from build123d import *

# Parameters (mm, degrees)
SKETCH_1_W          = 95.45
SKETCH_1_H          = 35.35
SKETCH_1_R          = 2
EXTRUDE_1_DEPTH     = 5
SKETCH_2_R          = 2
CUT_EXTRUDE_1_DEPTH = 5


with BuildPart() as part:
    # 草图1 → 凸台-拉伸1 (new body)
    with BuildSketch(Plane(origin=(0, 0, 0), x_dir=(1, 0, 0), z_dir=(0, 1, 0))):
        with Locations((8.528940217, -2.479891304)):
            Rectangle(SKETCH_1_W, SKETCH_1_H)
        with Locations(Location((-31.196059783, 7.195108696, 0), (0, 0, 270))):
            Circle(SKETCH_1_R, mode=Mode.SUBTRACT)
        with Locations(Location((-31.196059783, -12.154891304, 0), (0, 0, 270))):
            Circle(SKETCH_1_R, mode=Mode.SUBTRACT)
        with Locations(Location((48.253940217, 7.195108696, 0), (0, 0, 270))):
            Circle(SKETCH_1_R, mode=Mode.SUBTRACT)
        with Locations(Location((48.253940217, -12.154891304, 0), (0, 0, 270))):
            Circle(SKETCH_1_R, mode=Mode.SUBTRACT)
    extrude(amount=EXTRUDE_1_DEPTH)

    # 草图2 → 切除-拉伸1 (cut)
    with BuildSketch(Plane(origin=(0, 5, 0), x_dir=(1, 0, 0), z_dir=(0, 1, 0))):
        with Locations(Location((-18.971059783, -2.735165491, 0), (0, 0, 270))):
            Circle(SKETCH_2_R)
        with Locations(Location((36.028940217, -2.735165491, 0), (0, 0, 270))):
            Circle(SKETCH_2_R)
    extrude(amount=-CUT_EXTRUDE_1_DEPTH, mode=Mode.SUBTRACT)


solid = part.part
Read the model definition and answer for the solid it produces. Units are mm, in the model's axes. Give positions to 0.01 mm unless a question says otherwise; leave off trailing zeros. Write each loop counter-clockwise with the first axis right and the second up, starting at its lowest first coordinate (ties: lowest second). Pieces come first, ordered by that corner, then holes. Notation, with made-up numbers: (78.5, 41) - (109.5, 41) arc R20 cw to (109.5, 74) - close; hole circle Ø3 at (-20.75, -22). An arc over 180 degrees is marked (long way). Use CSV: the item, a comma, the result in double quotes. Start each with the question number.
(1) Consider line 1 along X through (y, z) = (3.6, -7); line 2 along Z through (x, y) = (-31, 3.1); line 3 along X through (y, z) = (2.6, -8.5). Determine where each line is inside the solid, lowest interval first.
(2) Find section B-B (z = 13). Give the vertices of the cut face in (x, y), plus the area to 3 significant figures.
(3) Given P1, Ø2.5, axis at x = 48.25, z = 12.15, coming from the +Y side; P2, Ø5, axis at x = 48.25, z = -7.2, coming from the +Y side, each flat-ended and moving along its own axis, determine where each tip first touches the part or whether it passes through.
(4) Determine the mould class of faces 1 (the flat face through (8, 5, 2)), 2 (the cylindrical face through (-20.745, 2.535, 3.658)), 3 (the flat face through (56.254, 2, 3)) for opening direction X: +X half, -X half, draft (parallel to the pull), parting line (faces both ways), or undercut.
(5) Find section A-A (y = 1.85). Give the vertices of the cut face in (x, z), plus the area to 3 significant figures.
Findings below:
1,line 1,"-39.2 to -33.19, -29.21 to 46.26, 50.24 to 56.25"
1,line 2,"-15.2 to -9.19, -5.2 to 10.16, 14.15 to 20.15"
1,line 3,"-39.2 to -32.71, -29.68 to 46.74, 49.77 to 56.25"
2,outline,"(-39.2, 0) - (-33.01, 0) - (-33.01, 5) - (-39.2, 5) - close; (-29.38, 0) - (46.44, 0) - (46.44, 5) - (-29.38, 5) - close; (50.07, 0) - (56.25, 0) - (56.25, 5) - (50.07, 5) - close"
2,area,"441 mm2"
3,P1,"through"
3,P2,"y = 5"
4,face 1,"draft"
4,face 2,"undercut"
4,face 3,"+X half"
5,outline,"(-39.2, -15.2) - (56.25, -15.2) - (56.25, 20.15) - (-39.2, 20.15) - close; hole circle Ø4 at (-31.2, -7.2); hole circle Ø4 at (-31.2, 12.15); hole circle Ø4 at (-18.97, 2.74); hole circle Ø4 at (36.03, 2.74); hole circle Ø4 at (48.25, -7.2); hole circle Ø4 at (48.25, 12.15)"
5,area,"3,300 mm2"
